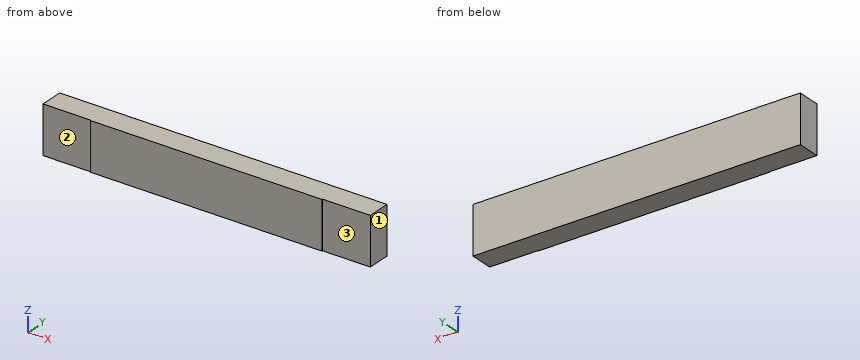
```python
from build123d import *

# Parameters (mm, degrees)
F0_W     = 609.6
F0_H     = 88.9
F1_DEPTH = 44.45
F2_W     = 88.9
F2_H     = 88.9
F3_DEPTH = 1.27
F4_DEPTH = 1.27


with BuildPart() as f1:
    # F0 (on Front) → F1 (new body)
    with BuildSketch(Plane.XZ):
        with Locations((-304.8, 44.45)):
            Rectangle(F0_W, F0_H)
    extrude(amount=F1_DEPTH)

    # F2 (on face) → F3 (cut)
    with BuildSketch(Plane.XZ.offset(44.45)):
        with Locations((-565.15, 44.45)):
            Rectangle(F2_W, F2_H)
    extrude(amount=-F3_DEPTH, mode=Mode.SUBTRACT)

    # F2 (on face) → F4 (cut)
    with BuildSketch(Plane.XZ.offset(44.45)):
        with Locations((-44.45, 44.45)):
            Rectangle(F2_W, F2_H)
    extrude(amount=-F4_DEPTH, mode=Mode.SUBTRACT)


solid = f1.part
```
Can you work these out from the model? Positions are in its coordinate system, mm. Face numbers are marked on the shaded views. A direction names the side the tool comes from. Round coordinates to 2 decimals unless told otherwise and drop trailing zeros. Order: outer loops, then holes, each group sorted by start corner. A loop starts at its lowest first (then second) coordinate and runs counter-clockwise, first axis right, second up.
(1) If we section it at A-A (x = -41): Please give me the cut outline in (y, z).
Results are:
outline: (-43.18, 0) - (0, 0) - (0, 88.9) - (-43.18, 88.9) - close
(2) On a 3-axis mill with a long thin cutter (end or side, diameter ignored), from which of +Z, -Z, +X, -X, +Y, -Y can I reach the whole of each face in a straight line? I mean the marked faces 1, 2 and 3. Say none if no direction works.
Results are:
face 1: +Z, -Z, +X, +Y, -Y
face 2: +Z, -Z, -X, -Y
face 3: +Z, -Z, +X, -Y
(3) I'm going to push flat-ended pins straight in: pin 1 (1.4 mm diameter, centred on y = -44, z = 57, fed in from +X); pin 2 (0.6 mm diameter, centred on y = -44, z = 42, fed in from -X). Where does each tip first touch, or does it pass through?
Results are:
pin 1: stops at x = -88.9
pin 2: stops at x = -520.7
(4) If I drill on L1, parallel to Y at x = -37.5, z = 34, over which ranges is the centre line in solid material (lowest first)?
Results are:
L1: y = -43.18 to 0
